Verification items for the finished model (mm, model axes). Give positions to 0.01 mm unless a question says otherwise; leave off trailing zeros. Write each loop counter-clockwise with the first axis right and the second up, starting at its lowest first coordinate (ties: lowest second). Pieces come first, ordered by that corner, then holes.
from build123d import *

# Parameters (mm, degrees)
ESQUISSE1_R      = 6.5
ESQUISSE1_R_2    = 3
EXTRUSION1_DEPTH = 2.5
ESQUISSE2_R      = 2.5
EXTRUSION2_DEPTH = 2.5
EXTRUSION3_DEPTH = 1.75
CONG_1_R         = 0.2


with BuildPart() as part:
    # Esquisse1 → Extrusion1 (new body, symmetric)
    with BuildSketch(Plane.XY):
        Circle(ESQUISSE1_R)
        Circle(ESQUISSE1_R_2, mode=Mode.SUBTRACT)
    extrude(amount=EXTRUSION1_DEPTH, both=True)



with BuildPart() as body_2:
    # Esquisse2 → Extrusion2 (new body, symmetric)
    with BuildSketch(Plane(origin=(0, 0, 0), x_dir=(0, 0, -1), z_dir=(1, 0, 0))):
        with Locations((0, 10)):
            Circle(ESQUISSE2_R)
    extrude(amount=EXTRUSION2_DEPTH, both=True)


with BuildPart() as part_1:
    add(part.part)

    add(body_2.part)  # Extrusion3 merges body 2
    # Esquisse3 → Extrusion3 (add, symmetric)
    with BuildSketch(Plane.XY):
        with BuildLine():
            Line((-2.5, 10), (2.5, 10))
            Line((2.5, 10), (2.5, 6))
            ThreePointArc((2.5, 6), (0, 6.5), (-2.5, 6))
            Line((-2.5, 6), (-2.5, 10))
        make_face()
    extrude(amount=EXTRUSION3_DEPTH, both=True)

    # Congé1
    cong_1_edges = [part_1.edges().sort_by_distance(p)[0] for p in [
        (0, 6.5, -1.75),
        (-2.5, 6, 0),
        (2.5, 7.107321446, -1.75),
        (2.5, 6, 0),
        (0, 6.5, 1.75),
        (2.5, 7.107321446, 1.75),
        (-6.5, 0, -2.5),
        (-2.5, 7.107321446, -1.75),
        (0, 8.214642893, -1.75),
        (-2.5, 7.107321446, 1.75),
        (0, 8.214642893, 1.75),
        (-2.5, 12.5, 0),
        (2.5, 12.5, 0),
        (-6.5, 0, 2.5),
    ]]
    fillet(cong_1_edges, radius=CONG_1_R)


solid = part_1.part
Item 1: Sectioned sample at A-A on z = 0. Record the cut outline in (x, y).
Answer key:
outline: (-2.62, 5.95) arc R6.5 ccw (long way) to (2.62, 5.95) arc R0.2 cw to (2.5, 6.13) - (2.5, 12.3) arc R0.2 ccw to (2.3, 12.5) - (-2.3, 12.5) arc R0.2 ccw to (-2.5, 12.3) - (-2.5, 6.13) arc R0.2 cw to start; hole circle Ø6 at (0, 0)
Item 2: Release check for a two-part mould opening along X. For faces 1 (the face through (-2.5, 9, 0)), 2 (the face through (2.5, 9, 0)), 3 (the face through (0, 7, -1.75)), 4 (the face through (-3, 0, 0)) record: released by +X, released by -X, zero draft, split by the parting line, or undercut.
Answer key:
face 1: released by -X
face 2: released by +X
face 3: zero draft
face 4: undercut
Item 3: Scan lines: line 1 along Y through (x, z) = (-1.5, -1.8); line 2 along X through (y, z) = (7, 1.3); line 3 along Y through (x, z) = (0, 0.35). Record each from-to range of solid material in increasing order.
Answer key:
line 1: y = -6.32 to -2.6, 2.6 to 6.39, 8.26 to 11.73
line 2: x = -2.5 to 2.5
line 3: y = -6.5 to -3, 3 to 12.48
Item 4: Depth check by flat-ended pin: pin 1 (1.4 mm diameter, centred on y = 9.5, z = -0.5, fed in from -X); pin 2 (1.4 mm diameter, centred on y = 9, z = -0.5, fed in from +X). Enter the tip coordinate at first touch or a pass-through.
Answer key:
pin 1: stops at x = -2.5
pin 2: stops at x = 2.5
Item 5: Sectioned sample at B-B on x = 0. Record the cut outline in (y, z).
Answer key:
outline: (-6.5, -2.3) arc R0.2 ccw to (-6.3, -2.5) - (-3, -2.5) - (-3, 2.5) - (-6.3, 2.5) arc R0.2 ccw to (-6.5, 2.3) - close; (3, -2.5) - (6.3, -2.5) arc R0.2 ccw to (6.5, -2.3) - (6.5, -1.95) arc R0.2 cw to (6.7, -1.75) - (8.13, -1.75) arc R0.2 cw to (8.27, -1.81) arc R2.5 ccw (long way) to (8.27, 1.81) arc R0.2 cw to (8.13, 1.75) - (6.7, 1.75) arc R0.2 cw to (6.5, 1.95) - (6.5, 2.3) arc R0.2 ccw to (6.3, 2.5) - (3, 2.5) - close
Item 6: Sectioned sample at C-C on y = 10. Record the cut outline in (x, z).
Answer key:
outline: (-2.5, -2.3) arc R0.2 ccw to (-2.3, -2.5) - (2.3, -2.5) arc R0.2 ccw to (2.5, -2.3) - (2.5, 2.3) arc R0.2 ccw to (2.3, 2.5) - (-2.3, 2.5) arc R0.2 ccw to (-2.5, 2.3) - close
